Verification items for the finished model (mm, model axes). Coordinates: 2 decimals unless noted, no trailing zeros. Loops run counter-clockwise (first coordinate to the right, second up) from the corner with the lowest first, then second, coordinate; pieces in that order, holes last.
Q1. Material ranges on probe 1 along Z at (x, y) = (29, -1.4); probe 2 along X at (y, z) = (-1.9, 8); probe 3 along Z at (x, y) = (35.5, -0.8), recorded low to high.
Q2. Sectioned sample at D-D (z = 32). Enter the section's corners in (x, y), then the cut area to 3 significant figures.
Q3. Sectioned sample at C-C (y = -1.8). Count the separate pieces of the cut face and the enclosed holes in it, then the cut area to 3 significant figures.
Q4. Sectioned sample at A-A (z = -8). Enter the section's corners in (x, y), then the cut area to 3 significant figures.
Q5. Sectioned sample at B-B (x = -29). Enter the section's corners in (y, z), then the cut area to 3 significant figures.
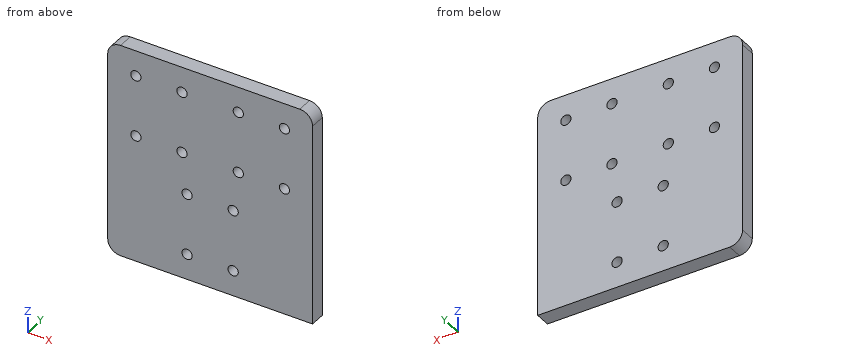
```python
from build123d import *

# Parameters (mm, degrees)
F0_W     = 80
F0_H     = 84
F0_W_2   = 30
F0_H_2   = 34
F0_W_3   = 18
F0_H_3   = 24
F1_DEPTH = 6
F2_D     = 4
F3_R     = 5


with BuildPart() as f1:
    # F0 (on Front) → F1 (new body)
    with BuildSketch(Plane.XZ):
        Rectangle(F0_W, F0_H)
        with Locations((0, -20)):
            Rectangle(F0_W_2, F0_H_2, mode=Mode.SUBTRACT)
        with Locations((-20, 20)):
            Rectangle(F0_W_2, F0_H_2, mode=Mode.SUBTRACT)
        with Locations((20, 20)):
            Rectangle(F0_W_2, F0_H_2, mode=Mode.SUBTRACT)
        with Locations((-20, 20)):
            Rectangle(F0_W_2, F0_H_2)
        with Locations((-20, 20)):
            Rectangle(F0_W_3, F0_H_3, mode=Mode.SUBTRACT)
        with Locations((20, 20)):
            Rectangle(F0_W_2, F0_H_2)
        with Locations((20, 20)):
            Rectangle(F0_W_3, F0_H_3, mode=Mode.SUBTRACT)
        with Locations((0, -20)):
            Rectangle(F0_W_2, F0_H_2)
        with Locations((0, -20)):
            Rectangle(F0_W_3, F0_H_3, mode=Mode.SUBTRACT)
        with Locations((-20, 20)):
            Rectangle(F0_W_3, F0_H_3)
        with Locations((20, 20)):
            Rectangle(F0_W_3, F0_H_3)
        with Locations((0, -20)):
            Rectangle(F0_W_3, F0_H_3)
    extrude(amount=F1_DEPTH)

    # F2 (through all)
    with Locations(Plane(origin=(0, 0, 0), x_dir=(1, 0, 0), z_dir=(0, 1, 0))):
        with Locations((-29, -32), (-11, -32), (-29, -8), (-11, -8), (11, -32), (29, -32), (29, -8), (11, -8), (9, 8), (-9, 8), (-9, 32), (9, 32)):
            Hole(F2_D / 2)

    # F3
    f3_edges = [f1.edges().sort_by_distance(p)[0] for p in [
        (-40, -3, 42),
        (-40, -3, -42),
        (40, -3, 42),
    ]]
    fillet(f3_edges, radius=F3_R)


solid = f1.part
```
Geometry check:
1. probe 1: z = -42 to 6, 10 to 30, 34 to 42
1. probe 2: x = -40 to -31, -27 to -13, -9 to 9, 13 to 27, 31 to 40
1. probe 3: z = -42 to 41.97
2. outline: (-40, -6) - (-31, -6) - (-31, 0) - (-40, 0) - close; (-27, -6) - (-13, -6) - (-13, 0) - (-27, 0) - close; (-9, -6) - (9, -6) - (9, 0) - (-9, 0) - close; (13, -6) - (27, -6) - (27, 0) - (13, 0) - close; (31, -6) - (40, -6) - (40, 0) - (31, 0) - close
2. area: 384 mm2
3. separate pieces: 1
3. enclosed holes: 12
3. area: 6,550 mm2
4. outline: (-40, -6) - (-11, -6) - (-11, 0) - (-40, 0) - close; (-7, -6) - (7, -6) - (7, 0) - (-7, 0) - close; (11, -6) - (40, -6) - (40, 0) - (11, 0) - close
4. area: 432 mm2
5. outline: (-6, -42) - (0, -42) - (0, 6) - (-6, 6) - close; (-6, 10) - (0, 10) - (0, 30) - (-6, 30) - close; (-6, 34) - (0, 34) - (0, 42) - (-6, 42) - close
5. area: 456 mm2
